from build123d import *

# Parameters (mm, degrees)
SKETCH_1_R          = 4.04
SKETCH_1_R_2        = 1.75
SKETCH_1_R_3        = 2.1
EXTRUDE_1_DEPTH     = 16
SKETCH_2_W          = 42
SKETCH_2_H          = 10
SKETCH_2_W_2        = 41
CUT_EXTRUDE_1_DEPTH = 218.479309361
SKETCH_3_R          = 4.1
A_0P1_DEPTH         = 0.1
B_0P1_START         = -0.1
SKETCH_4_R          = 4.1
B_0P1_DEPTH         = 0.1
SKETCH_5_R          = 6.25
A_0P1_2_DEPTH       = 0.1
SKETCH_6_R          = 6.25
B_0P1_2_DEPTH       = 0.1


with BuildPart() as part:
    # 草图1 → 凸台-拉伸1 (new body)
    with BuildSketch(Plane.XY):
        with BuildLine():
            Line((0, 6.5), (210, 6.5))
            ThreePointArc((210, 6.5), (216.5, 0), (210, -6.5))
            Line((210, -6.5), (0, -6.5))
            ThreePointArc((0, -6.5), (-6.5, 0), (0, 6.5))
        make_face()
        Circle(SKETCH_1_R, mode=Mode.SUBTRACT)
        with Locations((100, 0)):
            Circle(SKETCH_1_R_2, mode=Mode.SUBTRACT)
        with Locations((210, 0)):
            Circle(SKETCH_1_R_3, mode=Mode.SUBTRACT)
        with Locations((52, 0)):
            Circle(SKETCH_1_R_2, mode=Mode.SUBTRACT)
    extrude(amount=-EXTRUDE_1_DEPTH)

    # 草图2 → 切除-拉伸1 (cut, through all)
    with BuildSketch(Plane.XZ.offset(6.5)):
        Polygon((148.5, -3), (153.5, -3), (216.5, -3), (216.5, -13), (153.5, -13), (148.5, -13), (105.5, -13), (105.5, -3), align=None)
        with Locations((27.5, -8)):
            Rectangle(SKETCH_2_W, SKETCH_2_H)
        with Locations((77, -8)):
            Rectangle(SKETCH_2_W_2, SKETCH_2_H)
    extrude(amount=-CUT_EXTRUDE_1_DEPTH, mode=Mode.SUBTRACT)

    # 草图3 → A__0p1 (cut)
    with BuildSketch(Plane.XY):
        with Locations((210, 0)):
            Circle(SKETCH_3_R)
    extrude(amount=-A_0P1_DEPTH, mode=Mode.SUBTRACT)

    # 草图4 → B__0p1 (cut)
    with BuildSketch(Plane(origin=(0, 0, -16), x_dir=(-1, 0, 0), z_dir=(0, 0, -1)).offset(B_0P1_START)):
        with Locations(Location((-210, 0, 0), (0, 0, 180))):
            Circle(SKETCH_4_R)
    extrude(amount=B_0P1_DEPTH, mode=Mode.SUBTRACT)

    # 草图5 → A__0p1 2 (cut)
    with BuildSketch(Plane(origin=(0, 0, -3), x_dir=(-1, 0, 0), z_dir=(0, 0, -1))):
        with Locations((-210, 0)):
            Circle(SKETCH_5_R)
    extrude(amount=-A_0P1_2_DEPTH, mode=Mode.SUBTRACT)

    # 草图6 → B__0p1 2 (cut)
    with BuildSketch(Plane.XY.offset(-13).offset(B_0P1_START)):
        with Locations(Location((210, 0, 0), (0, 0, 180))):
            Circle(SKETCH_6_R)
    extrude(amount=B_0P1_2_DEPTH, mode=Mode.SUBTRACT)


solid = part.part
For this review, take the finished solid that the model builds, in its own axes (mm). A direction names the side the tool comes from. Give positions to 0.01 mm unless a question says otherwise; leave off trailing zeros. Loops run counter-clockwise (first coordinate to the right, second up) from the corner with the lowest first, then second, coordinate; pieces in that order, holes last.
Item 1: For line 1 along Z through (x, y) = (45, -4); line 2 along X through (y, z) = (-0.25, -9); line 3 along X through (y, z) = (6, -6.5), list the stretches that pass through material, from the lowest coordinate up.
Item 2: Insertion check: pin 1 (6 mm diameter, centred on y = 3, z = -11, fed in from +X); pin 2 (5.5 mm diameter, centred on x = 210, y = 0, fed in from -Z); pin 3 (2.5 mm diameter, centred on x = 210, y = -1.5, fed in from +Z). Each pin has a flat end and moves straight along its axis. Give the tip position at first contact, or say it passes through.
Item 3: Take a section at B-B, the plane x = 93. State the section outline as (y, z) points.
Item 4: Tool access review of faces 1 (the cylindrical face through (3.853, 1.214, -7.888)), 2 (the flat face through (48.5, 0, -8)): name each direction out of +Z, -Z, +X, -X, +Y, -Y from which nothing blocks a thin tool from reaching the whole face with its end or side.
Item 5: Draft analysis for pull direction Y (two halves, no side actions). For faces 3 (the flat face through (107, 0, 0)), 4 (the cylindrical face through (212.003, 0.631, -1.48)), 5 (the cylindrical face through (-6.5, -0.1, -7.9)), state which applies: +Y half, -Y half, draft (parallel to the pull), parting line (faces both ways), or undercut.
Item 6: Take a section at A-A, the plane z = -9. State the section outline as (x, y) points, and give its area (3 significant figures).
Calculated:
1. line 1: z = -16 to -13, -3 to 0
1. line 2: x = -6.5 to -4.03, 4.03 to 6.5, 48.5 to 50.27, 53.73 to 56.5, 97.5 to 98.27, 101.73 to 105.5
1. line 3: x = -2.5 to 6.5, 48.5 to 56.5, 97.5 to 105.5
2. pin 1: stops at x = 216.45
2. pin 2: stops at z = -15.9
2. pin 3: stops at z = -0.1
3. outline: (-6.5, -16) - (6.5, -16) - (6.5, -13) - (-6.5, -13) - close; (-6.5, -3) - (6.5, -3) - (6.5, 0) - (-6.5, 0) - close
4. face 1: +Z, -Z
4. face 2: +Y, -Y
5. face 3: draft
5. face 4: undercut
5. face 5: parting line
6. outline: (0, -6.5) - (6.5, -6.5) - (6.5, 6.5) - (0, 6.5) arc R6.5 ccw to start; (48.5, -6.5) - (56.5, -6.5) - (56.5, 6.5) - (48.5, 6.5) - close; (97.5, -6.5) - (105.5, -6.5) - (105.5, 6.5) - (97.5, 6.5) - close; hole circle Ø8.08 at (0, 0); hole circle Ø3.5 at (52, 0); hole circle Ø3.5 at (100, 0)
6. area: 288 mm2
